```python
from build123d import *

# Parameters (mm, degrees)
SKETCH1_R           = 80
BOSS_EXTRUDE1_DEPTH = 1.5875
SKETCH2_R           = 1
SKETCH2_R_2         = 0.85
CUT_EXTRUDE2_DEPTH  = 114.181626711


with BuildPart() as part:
    # Sketch1 → Boss-Extrude1 (new, symmetric)
    with BuildSketch(Plane(origin=(0, 0, 0), x_dir=(1, 0, 0), z_dir=(0, 1, 0))):
        with Locations(Location((0, 0, 0), (0, 0, 270))):
            Circle(SKETCH1_R)
    extrude(amount=BOSS_EXTRUDE1_DEPTH, both=True)

    # Sketch2 → Cut-Extrude2 (cut, through all)
    # profile 1 of 8: a face of its own
    with BuildSketch(Plane.XZ.offset(1.5875)):
        with Locations(Location((16.45, 0, 0), (0, 0, 270))):
            Circle(SKETCH2_R)
        with Locations((16.45, 0)):
            Circle(SKETCH2_R_2, mode=Mode.SUBTRACT)
    # profile 2 of 8: a face of its own
    with BuildSketch(Plane.XZ.offset(1.5875)):
        with Locations((16.45, 0)):
            Circle(SKETCH2_R_2)
    # profile 3 of 8: a face of its own
    with BuildSketch(Plane.XZ.offset(1.5875)):
        with Locations(Location((0, -16.45, 0), (0, 0, 270))):
            Circle(SKETCH2_R)
        with Locations((0, -16.45)):
            Circle(SKETCH2_R_2, mode=Mode.SUBTRACT)
    # profile 4 of 8: a face of its own
    with BuildSketch(Plane.XZ.offset(1.5875)):
        with Locations((0, -16.45)):
            Circle(SKETCH2_R_2)
    # profile 5 of 8: a face of its own
    with BuildSketch(Plane.XZ.offset(1.5875)):
        with Locations(Location((-16.45, 0, 0), (0, 0, 270))):
            Circle(SKETCH2_R)
        with Locations((-16.45, 0)):
            Circle(SKETCH2_R_2, mode=Mode.SUBTRACT)
    # profile 6 of 8: a face of its own
    with BuildSketch(Plane.XZ.offset(1.5875)):
        with Locations((-16.45, 0)):
            Circle(SKETCH2_R_2)
    # profile 7 of 8: a face of its own
    with BuildSketch(Plane.XZ.offset(1.5875)):
        with Locations(Location((0, 16.45, 0), (0, 0, 270))):
            Circle(SKETCH2_R)
        with Locations((0, 16.45)):
            Circle(SKETCH2_R_2, mode=Mode.SUBTRACT)
    # profile 8 of 8: a face of its own
    with BuildSketch(Plane.XZ.offset(1.5875)):
        with Locations((0, 16.45)):
            Circle(SKETCH2_R_2)
    extrude(amount=-CUT_EXTRUDE2_DEPTH, mode=Mode.SUBTRACT)


solid = part.part
```
The model under review builds one solid part; all positions refer to its coordinate system, in mm. Round coordinates to 2 decimals unless told otherwise and drop trailing zeros. Order: outer loops, then holes, each group sorted by start corner. A loop starts at its lowest first (then second) coordinate and runs counter-clockwise, first axis right, second up.
(1) For P1, Ø1.6, axis at x = 0, z = 16.45, coming from the +Y side; P2, Ø1, axis at y = 1, z = -13.5, coming from the +X side, all flat-tipped, find the tip position at first contact; note any pin that passes through.
Working result:
P1: passes through
P2: stops at x = 78.94
(2) Take a section at B-B, the plane x = -64. State the section outline as (y, z) points.
Working result:
outline: (-1.59, -48) - (1.59, -48) - (1.59, 48) - (-1.59, 48) - close
(3) Take a section at A-A, the plane y = -1.1. State the section outline as (x, z) points.
Working result:
outline: circle Ø160 at (0, 0); hole circle Ø2 at (-16.45, 0); hole circle Ø2 at (0, -16.45); hole circle Ø2 at (0, 16.45); hole circle Ø2 at (16.45, 0)
(4) Take a section at C-C, the plane z = 68. State the section outline as (x, y) points.
Working result:
outline: (-42.14, -1.59) - (42.14, -1.59) - (42.14, 1.59) - (-42.14, 1.59) - close
(5) Wall thickness on L1, parallel to X at y = -0.4, z = 0; L2, parallel to X at y = -0.65, z = -16.45; L3, parallel to Z at x = -40, y = -0.25: over which ranges is each line inside the solid? List them lowest first.
Working result:
L1: x = -80 to -17.45, -15.45 to 15.45, 17.45 to 80
L2: x = -78.29 to -1, 1 to 78.29
L3: z = -69.28 to 69.28
